Build history of the part. All positions in model axes, mm. Round coordinates to 2 decimals unless told otherwise and drop trailing zeros. Use a Markdown table: item, result.
from build123d import *

# Parameters (mm, degrees)
F0_W     = 38.1
F0_H     = 381
F1_DEPTH = 6.35
F2_R     = 3.175
F3_DEPTH = 6.351
F4_R     = 1.5875
F5_DEPTH = 3.175
F6_R     = 1.473365
F6_R_2   = 1.414723
F7_DEPTH = 3.175


with BuildPart() as f1:
    # F0 (on Front) → F1 (new body)
    with BuildSketch(Plane.XZ):
        Rectangle(F0_W, F0_H)
    extrude(amount=F1_DEPTH)

    # F2 (on face) → F3 (cut, through all)
    with BuildSketch(Plane.XZ.offset(6.35)):
        with Locations((0, -85.725)):
            Circle(F2_R)
        with Locations((0, -60.325)):
            Circle(F2_R)
        with Locations((0, -34.925)):
            Circle(F2_R)
        with Locations((0, -9.525)):
            Circle(F2_R)
        with Locations((0, 15.875)):
            Circle(F2_R)
        with Locations((0, 41.275)):
            Circle(F2_R)
        with Locations((0, 66.675)):
            Circle(F2_R)
        with Locations((0, 92.075)):
            Circle(F2_R)
        with Locations((0, 117.475)):
            Circle(F2_R)
        with Locations((0, 142.875)):
            Circle(F2_R)
        with Locations((0, 168.275)):
            Circle(F2_R)
    extrude(amount=-F3_DEPTH, mode=Mode.SUBTRACT)

    # F4 (on face) → F5 (cut)
    with BuildSketch(Plane.XZ.offset(6.35)):
        with Locations((-15.875, 187.325)):
            Circle(F4_R)
        with Locations((15.875, 187.325)):
            Circle(F4_R)
    extrude(amount=-F5_DEPTH, mode=Mode.SUBTRACT)

    # F6 (on face) → F7 (cut)
    with BuildSketch(Plane.XZ.offset(6.35)):
        with Locations((-15.875, -187.325)):
            Circle(F6_R)
        with Locations((15.875, -187.325)):
            Circle(F6_R_2)
    extrude(amount=-F7_DEPTH, mode=Mode.SUBTRACT)


solid = f1.part
Q1. Cut at A-A on y = -1. Count the separate pieces of the cut face and the enclosed holes in it, and give its area (3 significant figures).
Response values:
| item | result |
|---|---|
| separate pieces | 1 |
| enclosed holes | 11 |
| area | 14,200 mm2 |
Q2. Two-plate mould, pull along X, no slides. Class faces 1 (the flat face through (0, -6.35, 3)), 2 (the flat face through (19.05, -3, -3)), 3 (the cylindrical face through (-0.413, -3.219, 19.023)), 4 (the cylindrical face through (-0.688, -3.219, -12.624)): +X half, -X half, draft (parallel to the pull), parting line (faces both ways), or undercut.
Response values:
| item | result |
|---|---|
| face 1 | draft |
| face 2 | +X half |
| face 3 | undercut |
| face 4 | undercut |
Q3. Drop flat-ended pins along their axis: P1, Ø5.5, axis at x = 0, z = 15.875, coming from the +Y side; P2, Ø0.9, axis at x = -15, z = -187, coming from the -Y side (3 decimals). Give the stop position or say it passes through.
Response values:
| item | result |
|---|---|
| P1 | passes through |
| P2 | stops at y = -3.175 |
